Part model, mm, in its own coordinate system. A direction names the side the tool comes from. Round coordinates to 2 decimals unless told otherwise and drop trailing zeros. Answer as CSV lines item,"result".
from build123d import *

# Parameters (mm, degrees)
ESBO_O1_R                = 7.5
ESBO_O1_R_2              = 1.6
RESSALTO_EXTRUS_O1_DEPTH = 4
FILETE2_R                = 10
FILETE3_R                = 5
FILETE4_R                = 2


with BuildPart() as part:
    # Esboço1 → Ressalto-extrusão1 (new body)
    with BuildSketch(Plane.XY):
        with BuildLine():
            Line((14.471901241, -53.5), (14.471901241, -66.5))
            Line((14.471901241, -66.5), (44.471901241, -66.5))
            Line((44.471901241, -66.5), (44.471901241, -47.5))
            Line((44.471901241, -47.5), (64.371965948, -47.5))
            ThreePointArc((64.371965948, -47.5), (80, 0), (64.371965948, 47.5))
            Line((64.371965948, 47.5), (44.471901241, 47.5))
            Line((44.471901241, 47.5), (44.471901241, 66.5))
            Line((44.471901241, 66.5), (14.471901241, 66.5))
            Line((14.471901241, 66.5), (14.471901241, 53.5))
            Line((14.471901241, 53.5), (-5.003543323, 53.5))
            Line((-5.003543323, 53.5), (-5.003543323, 47.5))
            Line((-5.003543323, 47.5), (-40.003543323, 47.5))
            Line((-40.003543323, 47.5), (-40.003543323, 53.5))
            Line((-40.003543323, 53.5), (-59.478987886, 53.5))
            ThreePointArc((-59.478987886, 53.5), (-65.948635083, 45.285511266), (-71.291651246, 36.297389198))
            Line((-71.291651246, 36.297389198), (-71.291651246, -36.297389198))
            ThreePointArc((-71.291651246, -36.297389198), (-65.948635083, -45.285511266), (-59.478987886, -53.5))
            Line((-59.478987886, -53.5), (-40.003543323, -53.5))
            Line((-40.003543323, -53.5), (-40.003543323, -47.5))
            Line((-40.003543323, -47.5), (-5.003543323, -47.5))
            Line((-5.003543323, -47.5), (-5.003543323, -53.5))
            Line((-5.003543323, -53.5), (14.471901241, -53.5))
        make_face()
        with Locations((-31.783703802, -35.29937921)):
            Circle(ESBO_O1_R, mode=Mode.SUBTRACT)
        with Locations((19.471901241, -57)):
            Circle(ESBO_O1_R_2, mode=Mode.SUBTRACT)
        with Locations((39.471901241, -57)):
            Circle(ESBO_O1_R_2, mode=Mode.SUBTRACT)
        with BuildLine():
            Line((25, -39.332538239), (-14.754798134, -39.332538239))
            ThreePointArc((-14.754798134, -39.332538239), (-14.287636143, -34.928412284), (-14.941054623, -30.548045856))
            Line((-14.941054623, -30.548045856), (0, -17.5))
            Line((0, -17.5), (25, -39.332538239))
        make_face(mode=Mode.SUBTRACT)
        with BuildLine():
            Line((-15, -10.684767074), (-24.807750727, -19.249890785))
            ThreePointArc((-24.807750727, -19.249890785), (-40.174599446, -19.942202702), (-49.058352164, -32.5))
            Line((-49.058352164, -32.5), (-56.291651246, -32.5))
            Line((-56.291651246, -32.5), (-56.291651246, 32.5))
            Line((-56.291651246, 32.5), (-39.980184035, 32.5))
            Line((-39.980184035, 32.5), (-15, 10.684767074))
            Line((-15, 10.684767074), (-15, -10.684767074))
        make_face(mode=Mode.SUBTRACT)
        with BuildLine():
            Line((49.058352164, 32.5), (56.291651246, 32.5))
            ThreePointArc((56.291651246, 32.5), (65, 0), (56.291651246, -32.5))
            Line((56.291651246, -32.5), (39.980184035, -32.5))
            Line((39.980184035, -32.5), (15, -10.684767074))
            Line((15, -10.684767074), (15, 10.684767074))
            Line((15, 10.684767074), (24.807750727, 19.249890785))
            ThreePointArc((24.807750727, 19.249890785), (40.174599446, 19.942202702), (49.058352164, 32.5))
        make_face(mode=Mode.SUBTRACT)
        with BuildLine():
            Line((0, 17.5), (-25, 39.332538239))
            Line((-25, 39.332538239), (14.754798134, 39.332538239))
            ThreePointArc((14.754798134, 39.332538239), (14.287636143, 34.928412284), (14.941054623, 30.548045856))
            Line((14.941054623, 30.548045856), (0, 17.5))
        make_face(mode=Mode.SUBTRACT)
        with Locations((19.471901241, 57)):
            Circle(ESBO_O1_R_2, mode=Mode.SUBTRACT)
        with Locations((39.471901241, 57)):
            Circle(ESBO_O1_R_2, mode=Mode.SUBTRACT)
        with Locations((31.783703802, 35.29937921)):
            Circle(ESBO_O1_R, mode=Mode.SUBTRACT)
    extrude(amount=RESSALTO_EXTRUS_O1_DEPTH)

    # Filete2
    filete2_edges = [part.edges().sort_by_distance(p)[0] for p in [
        (-71.291651246, -36.297389198, 2),
        (-71.291651246, 36.297389198, 2),
        (15, -10.684767074, 2),
        (39.980184035, -32.5, 2),
        (56.291651246, -32.5, 2),
        (-15, 10.684767074, 2),
        (-39.980184035, 32.5, 2),
        (-56.291651246, 32.5, 2),
    ]]
    fillet(filete2_edges, radius=FILETE2_R)

    # Filete3
    # the kernel refuses this fillet: 5 mm, written as the material it adds along each edge
    with BuildSketch(Plane(origin=(56.291651246, 32.5, 0), x_dir=(0.47930172295418866, -0.8776501913479802, 0), z_dir=(0, 0, 1))) as filete3_piece_1:
        with BuildLine():
            CenterArc((2.96720344, -4.998591114), FILETE3_R, 88.639806368, 62.720387264)
            Line((-1.421047517, -2.602082499), (0, 0))
            ThreePointArc((0, 0), (1.542945789, 0.018315517), (3.085891577, 0))
        make_face()
    extrude(amount=4)
    with BuildSketch(Plane(origin=(49.058352164, 32.5, 0), x_dir=(1, 0, 0), z_dir=(0, 0, 1))) as filete3_piece_2:
        with BuildLine():
            CenterArc((3.830319867, -5), FILETE3_R, 90, 69.718116788)
            ThreePointArc((-0.859673073, -3.26680462), (-0.35082821, -1.654193676), (0, 0))
            Line((0, 0), (3.830319867, 0))
        make_face()
    extrude(amount=4)
    with BuildSketch(Plane(origin=(24.807750727, 19.249890785, 0), x_dir=(0.9437647380510182, -0.3306177841730431, 0), z_dir=(0, 0, 1))) as filete3_piece_3:
        with BuildLine():
            CenterArc((2.919799374, -4.986661539), FILETE3_R, 94.186027535, 56.251011404)
            Line((-1.429270912, -2.519763153), (0, 0))
            ThreePointArc((0, 0), (1.277412226, -0.046684613), (2.554824452, 0))
        make_face()
    extrude(amount=4)
    with BuildSketch(Plane(origin=(15, 10.684767074, 0), x_dir=(0.7532103380208672, 0.6577797402615034, 0), z_dir=(0, 0, 1))) as filete3_piece_4:
        with BuildLine():
            CenterArc((FILETE3_R * 0.454348861751, -FILETE3_R), FILETE3_R, 90, 48.869237816)
            Line((-FILETE3_R * 0.29886147627, -FILETE3_R * 0.342220259738), (0, 0))
            Line((0, 0), (FILETE3_R * 0.454348861751, 0))
        make_face()
    extrude(amount=4)
    with BuildSketch(Plane(origin=(-15, -10.684767074, 0), x_dir=(0, 1, 0), z_dir=(0, 0, 1))) as filete3_piece_5:
        with BuildLine():
            CenterArc((FILETE3_R * 0.454348861751, FILETE3_R), FILETE3_R, 221.130762184, 48.869237816)
            Line((-FILETE3_R * 0.29886147627, FILETE3_R * 0.342220259738), (0, 0))
            Line((0, 0), (FILETE3_R * 0.454348861751, 0))
        make_face()
    extrude(amount=4)
    with BuildSketch(Plane(origin=(-24.807750727, -19.249890785, 0), x_dir=(0.7532103380209099, 0.6577797402614547, 0), z_dir=(0, 0, 1))) as filete3_piece_6:
        with BuildLine():
            CenterArc((2.896898633, 5), FILETE3_R, 213.748988596, 56.251011404)
            ThreePointArc((-1.260498463, 2.222222222), (-0.589642299, 1.13414435), (0, 0))
            Line((0, 0), (2.896898633, 0))
        make_face()
    extrude(amount=4)
    with BuildSketch(Plane(origin=(-49.058352164, -32.5, 0), x_dir=(0.2544898792174261, 0.9670754372725532, 0), z_dir=(0, 0, 1))) as filete3_piece_7:
        with BuildLine():
            CenterArc((3.860599546, 4.976657656), FILETE3_R, 194.74336021, 69.718116788)
            Line((-0.97477764, 3.70420826), (0, 0))
            ThreePointArc((0, 0), (1.689012301, 0.081698204), (3.378024603, 0))
        make_face()
    extrude(amount=4)
    with BuildSketch(Plane(origin=(14.754798134, 39.332538239, 0), x_dir=(-0.09464454898712658, -0.9955111296952049, 0), z_dir=(0, 0, 1))) as filete3_piece_8:
        with BuildLine():
            CenterArc((5.493397952, -4.952623325), FILETE3_R, 97.893660423, 87.537201367)
            Line((0.515842303, -5.42584607), (0, 0))
            ThreePointArc((0, 0), (2.403361604, -0.165818364), (4.806723208, 0))
        make_face()
    extrude(amount=4)
    with BuildSketch(Plane(origin=(0, 17.5, 0), x_dir=(0.7532103380208671, 0.6577797402615035, 0), z_dir=(0, 0, 1)), Plane(origin=(0, -17.5, 0), x_dir=(-0.7532103380208676, -0.6577797402615031, 0), z_dir=(0, 0, 1))) as filete3_piece_9:
        with BuildLine():
            CenterArc((FILETE3_R * 0.873301529543, FILETE3_R), FILETE3_R, 187.738475632, 82.261524368)
            Line((-FILETE3_R * 0.117591471468, FILETE3_R * 0.865348373397), (0, 0))
            Line((0, 0), (FILETE3_R * 0.873301529543, 0))
        make_face()
    extrude(amount=4)
    with BuildSketch(Plane(origin=(-14.754798134, -39.332538239, 0), x_dir=(1, 0, 0), z_dir=(0, 0, 1))) as filete3_piece_10:
        with BuildLine():
            CenterArc((5.450311812, 5), FILETE3_R, 182.462798633, 87.537201367)
            ThreePointArc((0.45493015, 4.785146451), (0.392539102, 2.376879421), (0, 0))
            Line((0, 0), (5.450311812, 0))
        make_face()
    extrude(amount=4)
    with BuildSketch(Plane(origin=(14.471901241, 53.5, 0), x_dir=(-1, 0, 0), z_dir=(0, 0, 1)), Plane(origin=(44.471901241, -47.5, 0), x_dir=(1, 0, 0), z_dir=(0, 0, 1)), Plane(origin=(44.471901241, 47.5, 0), x_dir=(0, 1, 0), z_dir=(0, 0, 1))) as filete3_piece_11:
        with BuildLine():
            CenterArc((FILETE3_R, -FILETE3_R), FILETE3_R, 90, 90)
            Line((0, -FILETE3_R), (0, 0))
            Line((0, 0), (FILETE3_R, 0))
        make_face()
    extrude(amount=4)
    with BuildSketch(Plane(origin=(14.471901241, -53.5, 0), x_dir=(-1, 0, 0), z_dir=(0, 0, 1)), Plane(origin=(-56.291651246, -32.5, 0), x_dir=(1, 0, 0), z_dir=(0, 0, 1))) as filete3_piece_12:
        with BuildLine():
            CenterArc((FILETE3_R, FILETE3_R), FILETE3_R, 180, 90)
            Line((0, FILETE3_R), (0, 0))
            Line((0, 0), (FILETE3_R, 0))
        make_face()
    extrude(amount=4)
    # the kernel refuses this fillet: 5 mm, written as the material it takes off along each edge
    with BuildSketch(Plane(origin=(14.471901241, -66.5, -12.5), x_dir=(0, 1, 0), z_dir=(0, 0, 1)), Plane(origin=(44.471901241, -66.5, -12.5), x_dir=(-1, 0, 0), z_dir=(0, 0, 1))) as filete3_2_piece_1:
        with BuildLine():
            CenterArc((FILETE3_R, -FILETE3_R), FILETE3_R, 90, 90)
            Line((0, -FILETE3_R), (0, 0))
            Line((0, 0), (FILETE3_R, 0))
        make_face()
    extrude(amount=29, mode=Mode.SUBTRACT)
    with BuildSketch(Plane(origin=(14.471901241, 66.5, -12.5), x_dir=(0, -1, 0), z_dir=(0, 0, 1)), Plane(origin=(44.471901241, 66.5, -12.5), x_dir=(-1, 0, 0), z_dir=(0, 0, 1))) as filete3_2_piece_2:
        with BuildLine():
            CenterArc((FILETE3_R, FILETE3_R), FILETE3_R, 180, 90)
            Line((0, FILETE3_R), (0, 0))
            Line((0, 0), (FILETE3_R, 0))
        make_face()
    extrude(amount=29, mode=Mode.SUBTRACT)

    # Filete4
    filete4_edges = [part.edges().sort_by_distance(p)[0] for p in [
        (-25, 39.332538239, 2),
        (25, -39.332538239, 2),
    ]]
    fillet(filete4_edges, radius=FILETE4_R)


solid = part.part
Q1. Saw through at A-A, the plane z = 3.35. Give the number of separate pieces and of enclosed holes in the cut face, then the cut area to 3 significant figures.
Geometry results:
separate pieces,"1"
enclosed holes,"10"
area,"9,890 mm2"
Q2. Drop flat-ended pins along their axis: P1, Ø2, axis at x = -54.5, z = 2, coming from the -Y side; P2, Ø2, axis at x = 11, z = 2.5, coming from the +Y side; P3, Ø2, axis at y = 50.5, z = 1.5, coming from the +X side; P4, Ø5, axis at x = 19.47, y = -57, coming from the +Z side. Give the stop position or say it passes through.
Geometry results:
P1,"y = -53.5"
P2,"y = 54.19"
P3,"x = 45.47"
P4,"z = 4"
Q3. Drill centre lines: line 1 along Y through (x, z) = (18.5, 0.65); line 2 along X through (y, z) = (-20, 0.9); line 3 along Y through (x, z) = (-34, 2.1). Where is each one in solid material? Low to high.
Geometry results:
line 1,"-66.4 to -58.27, -55.73 to -39.33, -33.66 to -13.74, 13.74 to 55.73, 58.27 to 66.4"
line 2,"-71.29 to -56.29, -40.28 to -2.81, 2.81 to 25.67, 61.85 to 77.46"
line 3,"-47.5 to -42.46, -28.13 to -17.94, 27.28 to 47.5"
Q4. Which spindle directions (+Z, -Z, +X, -X, +Y, -Y) get a long thin tool onto all of the face, cutting with end or side? Do faces 5 (the face through (-40.004, -51, 2)), 6 (the face through (-15.87, 10.22, 2.03)), 7 (the face through (3, -1, 4)). Say none if no direction does.
Geometry results:
face 5,"+Z, -Z, -Y"
face 6,"+Z, -Z"
face 7,"+Z, +X, -X, +Y, -Y"
Q5. Two-plate mould, pull along X, no slides. Class faces 1 (the face through (21, -56.52, 1.97)), 2 (the face through (16, 65.1, 2)), 3 (the face through (2, -53.5, 2)), 4 (the face through (79.997, -0.712, 1.972)): pulls with the +X half, pulls with the -X half, needs draft (parallel to the pull), parting line crosses it, or undercut.
Geometry results:
face 1,"undercut"
face 2,"pulls with the -X half"
face 3,"needs draft"
face 4,"pulls with the +X half"
